from build123d import *

# Parameters (mm, degrees)
SKETCH1_R             = 5.075
SKETCH1_R_2           = 1.6
SKETCH1_R_3           = 1.25
SKETCH1_R_4           = 2.1
SKETCH1_R_5           = 0.8
BOSS_EXTRUDE1_DEPTH   = 3.18
CHAMFER1_SIZE         = 2.5
CHAMFER1_SIZE2        = 4.998920521
FILLET2_R             = 3
CHAMFER2_SIZE         = 1.8
FILLET4_R             = 0.5
FILLET7_R             = 0.2
M3X0_5_TAPPED_HOLE1_D = 2.5
M2_TAPPED_HOLE1_D     = 1.6
FILLET8_R             = 0.3
CUT_EXTRUDE5_DEPTH    = 4


with BuildPart() as part:
    # Sketch1 → Boss-Extrude1 (new body)
    with BuildSketch(Plane(origin=(0, 0, 0), x_dir=(0, 0, -1), z_dir=(1, 0, 0))):
        Polygon((0, 0), (0, 34.275), (2, 36.275), (2, 65.31), (22, 65.31), (22, 45.31), (23.8, 45.31), (23.8, 26.21), (15.9, 26.21), (15.9, 15.26), (13.9, 15.26), (13.9, 13.26), (13.4, 13.26), (13.4, 11.86), (25.25, 11.86), (25.25, 6.86), (13.4, 6.86), (13.4, 0), align=None)
        with Locations(Location((7.075, 29.2, 0), (0, 0, 180))):
            Circle(SKETCH1_R, mode=Mode.SUBTRACT)
        with Locations(Location((7, 60.81, 0), (0, 0, 180))):
            Circle(SKETCH1_R_2, mode=Mode.SUBTRACT)
        with Locations(Location((17, 58.81, 0), (0, 0, 180))):
            Circle(SKETCH1_R_2, mode=Mode.SUBTRACT)
        with Locations(Location((22.4, 9.36, 0), (0, 0, 180))):
            Circle(SKETCH1_R_3, mode=Mode.SUBTRACT)
        with Locations(Location((16.4, 9.36, 0), (0, 0, 180))):
            Circle(SKETCH1_R_3, mode=Mode.SUBTRACT)
        with Locations(Location((3.15, 3.95, 0), (0, 0, 180))):
            Circle(SKETCH1_R_4, mode=Mode.SUBTRACT)
        with Locations(Location((3.15, 9.95, 0), (0, 0, 180))):
            Circle(SKETCH1_R_4, mode=Mode.SUBTRACT)
        with Locations(Location((10.15, 2.95, 0), (0, 0, 180))):
            Circle(SKETCH1_R_5, mode=Mode.SUBTRACT)
        with Locations(Location((3.15, 14.95, 0), (0, 0, 180))):
            Circle(SKETCH1_R_5, mode=Mode.SUBTRACT)
    extrude(amount=BOSS_EXTRUDE1_DEPTH)

    # Chamfer1
    chamfer1_edges = [part.edges().sort_by_distance(p)[0] for p in [
        (1.59, 0, -13.4),
    ]]
    chamfer1_side = [part.faces().sort_by_distance(p)[0] for p in [
        (1.59, 0, -6.7),
    ]]
    chamfer(chamfer1_edges, length=CHAMFER1_SIZE, length2=CHAMFER1_SIZE2, reference=chamfer1_side[0])

    # Fillet2
    fillet2_edges = [part.edges().sort_by_distance(p)[0] for p in [
        (1.59, 34.275, 0),
        (1.59, 36.275, -2),
    ]]
    fillet(fillet2_edges, radius=FILLET2_R)

    # Chamfer2
    chamfer2_edges = [part.edges().sort_by_distance(p)[0] for p in [
        (1.59, 65.31, -22),
        (1.59, 65.31, -2),
        (1.59, 45.31, -23.8),
    ]]
    chamfer(chamfer2_edges, length=CHAMFER2_SIZE - 0.0001)  # a hair under: the kernel refuses the full size

    # Fillet4
    fillet4_edges = [part.edges().sort_by_distance(p)[0] for p in [
        (1.59, 43.5101, -23.8),
        (1.59, 63.5101, -22),
        (1.59, 63.5101, -2),
        (1.59, 0, 0),
        (1.59, 4.998920521, -13.4),
    ]]
    fillet(fillet4_edges, radius=FILLET4_R)

    # Fillet7
    fillet7_edges = [part.edges().sort_by_distance(p)[0] for p in [
        (1.59, 13.26, -13.9),
        (1.59, 13.26, -13.4),
    ]]
    fillet(fillet7_edges, radius=FILLET7_R)

    # M3x0.5 Tapped Hole1 (through all)
    with Locations(Plane(origin=(3.18, 0, 0), x_dir=(0, 0, -1), z_dir=(1, 0, 0))):
        with Locations((16.4, 9.36), (22.4, 9.36)):
            Hole(M3X0_5_TAPPED_HOLE1_D / 2)

    # M2 Tapped Hole1 (through all)
    with Locations(Plane(origin=(0, 14.95, -3.15), x_dir=(0, 0, -1), z_dir=(-1, 0, 0))):
        with Locations((0, 0), (7, 12)):
            Hole(M2_TAPPED_HOLE1_D / 2)

    # Fillet8
    fillet8_edges = [part.edges().sort_by_distance(p)[0] for p in [
        (1.59, 15.26, -15.9),
        (1.59, 15.26, -13.9),
    ]]
    fillet(fillet8_edges, radius=FILLET8_R)

    # Sketch13 → Cut-Extrude5 (cut)
    with BuildSketch(Plane(origin=(3.18, 0, 0), x_dir=(0, 0, -1), z_dir=(1, 0, 0))):
        with BuildLine():
            Line((2, 42.81), (3.758141467, 42.81))
            ThreePointArc((3.758141467, 42.81), (19.460102, 45.31), (3.758141467, 47.81))
            Line((3.758141467, 47.81), (2, 47.81))
            Line((2, 47.81), (2, 42.81))
        make_face()
    extrude(amount=-CUT_EXTRUDE5_DEPTH, mode=Mode.SUBTRACT)


solid = part.part
The listing builds one solid part. Answer for the finished solid, in the listing's coordinates (mm). A direction names the side the tool comes from. Round coordinates to 2 decimals unless told otherwise and drop trailing zeros. Write each loop counter-clockwise with the first axis right and the second up, starting at its lowest first coordinate (ties: lowest second). Pieces come first, ordered by that corner, then holes. Notation, with made-up numbers: (-7, -32.75) - (48, -32.75) arc R14 cw to (48, -5.75) - close; hole circle Ø9 at (13.5, 62.25). An arc over 180 degrees is marked (long way). Use one line per item in the form item = value. Start each with the question number.
Item 1: A cutting plane is placed at D-D (x = 2.5). Give the number of separate pieces and of enclosed holes in the cut face, plus the area to 3 significant figures.
Item 2: Find the intervals of material crossed by line 1 (Y direction, x = 1.5, z = -7); line 2 (Y direction, x = 1.15, z = -17); line 3 (Y direction, x = 0.3, z = -18.25), in increasing order. Write a range as [from, to].
Item 3: Determine the mould class of faces 4 (the flat face through (2, 9, -25.25)), 5 (the flat face through (2, 6.86, -19)), 6 (the flat face through (1.57, 64.49, -2.98)), 7 (the flat face through (2, 47.81, -3)) for opening direction Y: +Y half, -Y half, draft (parallel to the pull), parting line (faces both ways), or undercut.
Item 4: A cutting plane is placed at B-B (z = -10.15). Write down the section's boundary in (x, y).
Item 5: A cutting plane is placed at A-A (y = 2.95). Write down the section's boundary in (x, z).
Item 6: A tool of negligible diameter and unlimited length cuts with its end or side. For faces 1 (the flat face through (2, 42.81, -3)), 2 (the flat face through (2, 0, -6)), 3 (the flat face through (2, 26.21, -20)), from which of +Z, -Z, +X, -X, +Y, -Y can it reach the whole face along a straight path? Write none if from no direction.
Item 7: A flat-ended cylindrical pin translates along its axis: pin 1 Ø1.6 at (x, y) = (1, 40) entering from +Z. Find the tip coordinate at first contact, or state that the pin passes through.
Item 8: A cutting plane is placed at C-C (y = 28). Write down the section's boundary in (x, z).
The answers:
q1.separate_pieces = 1
q1.enclosed_holes = 9
q1.area = 913 mm^2
q2.line_1 = [0, 24.13], [34.27, 38.58], [52.04, 59.21], [62.41, 65.31]
q2.line_2 = [6.86, 8.26], [10.46, 11.86], [26.21, 39.52], [51.1, 57.21], [60.41, 65.31]
q2.line_3 = [6.86, 11.86], [26.21, 41.07], [49.55, 57.81], [59.81, 65.31]
q3.face_4 = draft
q3.face_5 = -Y half
q3.face_6 = +Y half
q3.face_7 = undercut
q4.outline = (0, 0) - (3.18, 0) - (3.18, 2.15) - (0, 2.15) - close; (0, 3.75) - (3.18, 3.75) - (3.18, 25.16) - (0, 25.16) - close; (0, 33.24) - (3.18, 33.24) - (3.18, 37.36) - (0, 37.36) - close; (0, 53.26) - (3.18, 53.26) - (3.18, 65.31) - (0, 65.31) - close
q5.outline = (0, -12.38) - (3.18, -12.38) - (3.18, -10.95) - (0, -10.95) - close; (0, -9.35) - (3.18, -9.35) - (3.18, -5) - (0, -5) - close; (0, -1.3) - (3.18, -1.3) - (3.18, 0) - (0, 0) - close
q6.face_1 = +Z, +X, -X
q6.face_2 = +Z, -Z, +X, -X, -Y
q6.face_3 = -Z, +X, -X
q7.pin_1 = -2
q8.outline = (0, -23.8) - (3.18, -23.8) - (3.18, -12.01) - (0, -12.01) - close; (0, -2.14) - (3.18, -2.14) - (3.18, 0) - (0, 0) - close
